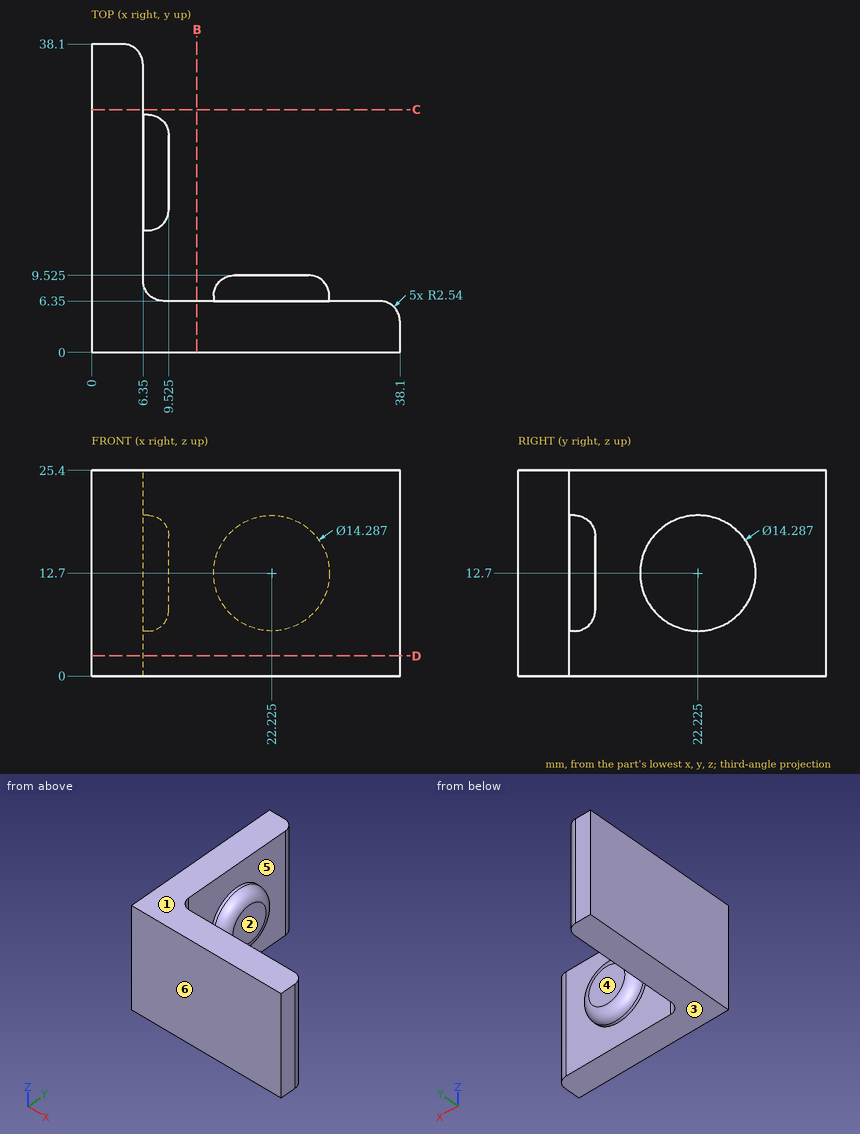
Geometry: see drawing. Coordinates: mm, zero at the bounding-box minimum. A direction names the side the tool comes from. Round coordinates to 2 decimals unless told otherwise and drop trailing zeros. Order: outer loops, then holes, each group sorted by start corner. A loop starts at its lowest first (then second) coordinate and runs counter-clockwise, first axis right, second up. Notation, with made-up numbers: (-1.75, -26.5) -> (6.25, -26.5) arc R18 cw to (6.25, -14.5) -> close; hole circle Ø11 at (-21, -32). An arc over 180 degrees is marked (long way). Answer as CSV lines item,"result".
Item 1: Section D-D, the plane z = 2.5. Return loops of the section in (x, y), plus the area to 3 significant figures.
A:
outline,"(0, 0) -> (38.1, 0) -> (38.1, 3.81) arc R2.54 ccw to (35.56, 6.35) -> (8.89, 6.35) arc R2.54 cw to (6.35, 8.89) -> (6.35, 35.56) arc R2.54 ccw to (3.81, 38.1) -> (0, 38.1) -> close"
area,"442 mm²"
Item 2: Line query: L1, parallel to X at y = 18.5, z = 5; L2, parallel to Y at x = 18, z = 14.5 (1 decimal). Output: solid intervals per line, ascending.
A:
L1,"0 to 6.35"
L2,"0 to 9.5"
Item 3: Pin query (flat end, axial travel): pin 1 Ø4 at (y, z) = (13, 5) entering from +X; pin 2 Ø10 at (x, z) = (20, 12) entering from +Y (1 decimal); pin 3 Ø1 at (x, z) = (22.5, 22) entering from +Y. Return the tip coordinate at first contact, or that it passes through.
A:
pin 1,"x = 6.35"
pin 2,"y = 9.5"
pin 3,"y = 6.35"
Item 4: Pull-direction query (Y, two-part tool) for the marked faces 3, 4, 5 and 6; classes: pulls with the +Y half, pulls with the -Y half, needs draft (parallel to the pull), parting line crosses it, or undercut.
A:
face 3,"needs draft"
face 4,"pulls with the +Y half"
face 5,"undercut"
face 6,"pulls with the -Y half"
Item 5: Reachability of the marked faces 1 and 2 from +Z, -Z, +X, -X, +Y, -Y: full face, straight path, thin tool, end or side. Return the list, or none.
A:
face 1,"+Z, +X, -X, +Y, -Y"
face 2,"+Z, -Z, +X, +Y"
Item 6: Section B-B, the plane x = 13. Return loops of the section in (y, z), plus the area to 3 significant figures.
A:
outline,"(0, 0) -> (6.35, 0) -> (6.35, 25.4) -> (0, 25.4) -> close"
area,"161 mm²"
